Verification items for this drawing (mm, ordinates from the low corner). A direction names the side the tool comes from. Coordinates: 2 decimals unless noted, no trailing zeros. Order: outer loops, then holes, each group sorted by start corner. A loop starts at its lowest first (then second) coordinate and runs counter-clockwise, first axis right, second up. Notation, with made-up numbers: M 61,64 L 115,64 A16 cw 115,89 Z; hole C 46.25,-24.5 d2. An arc over 180 degrees is marked long. One line per item, written item: value. Start each with the question number.
1) Go/stop test with flat-tipped pins: P1, Ø4, axis at x = 3.5, z = 7, coming from the +Y side; P2, Ø7.5, axis at x = 9, y = 16, coming from the -Z side. Record where each tip stops, or that it passes through.
2) Thickness scan on L1, parallel to Y at x = 16.75, z = 8.5; L2, parallel to Z at x = 18.5, y = 12.5; L3, parallel to Y at x = 17.5, z = 16.75. Record the ranges inside material, lowest first. Write a range as from..to.
3) Sectioned sample at B-B, the plane z = 9.75. Enter the section's corners in (x, y).
4) Sectioned sample at A-A, the plane x = 10. Enter the section's corners in (y, z).
5) Access from +Z, -Z, +X, -X, +Y, -Y to the whole of each face (thin tool, end or side, straight path). Record for the marked faces 1 and 2.
6) Sectioned sample at D-D, the plane z = 19. Enter the section's corners in (x, y).
7) Sectioned sample at C-C, the plane y = 9.75. Enter the section's corners in (x, z), then the cut area to 3 significant figures.
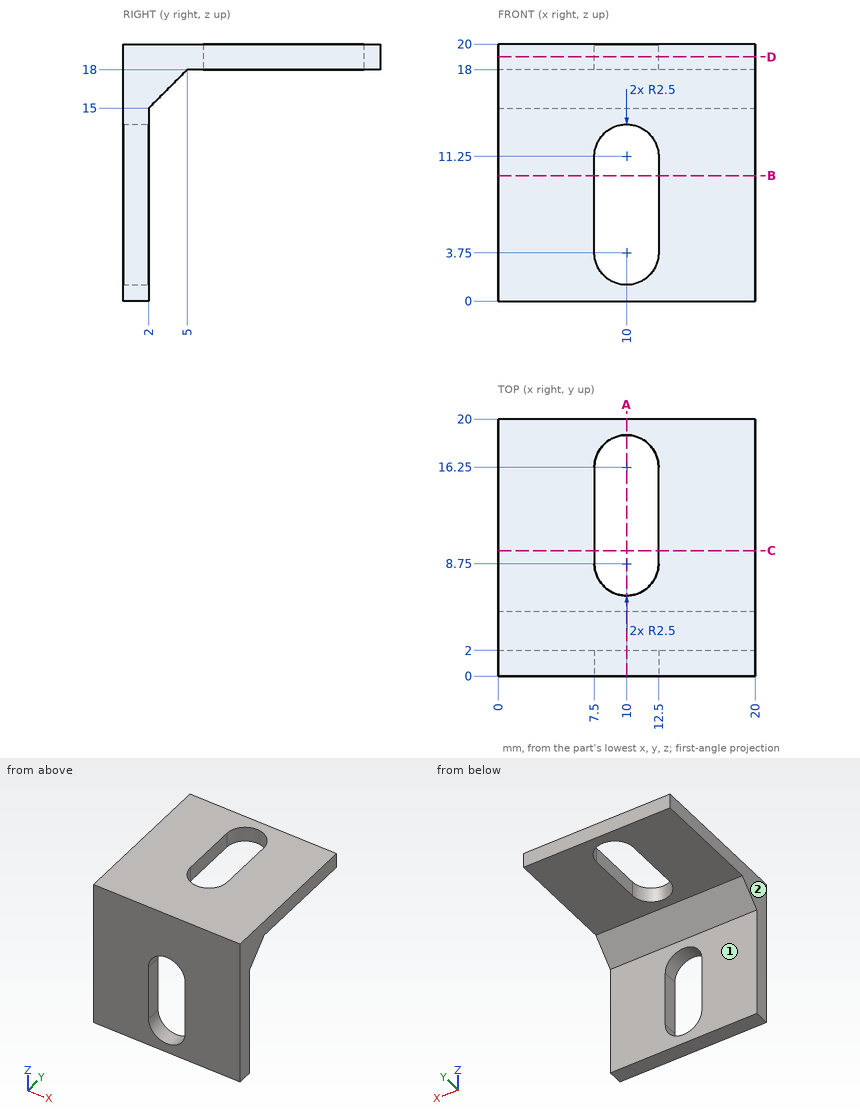
Final values:
1. P1: stops at y = 2
1. P2: stops at z = 18
2. L1: y = 0..2
2. L2: z = 18..20
2. L3: y = 0..3.75
3. outline: M 0,0 L 7.5,0 L 7.5,2 L 0,2 Z; M 12.5,0 L 20,0 L 20,2 L 12.5,2 Z
4. outline: M 0,0 L 2,0 L 2,1.25 L 0,1.25 Z; M 0,13.75 L 2,13.75 L 2,15 L 5,18 L 6.25,18 L 6.25,20 L 0,20 Z; M 18.75,18 L 20,18 L 20,20 L 18.75,20 Z
5. face 1: -Z, +X, -X, +Y
5. face 2: +Z, -Z, -X, +Y, -Y
6. outline: M 0,0 L 20,0 L 20,20 L 0,20 Z; hole M 7.5,8.75 A2.5 ccw 12.5,8.75 L 12.5,16.25 A2.5 ccw 7.5,16.25 Z
7. outline: M 0,18 L 7.5,18 L 7.5,20 L 0,20 Z; M 12.5,18 L 20,18 L 20,20 L 12.5,20 Z
7. area: 30.0 mm^2
